Build history of the part. All positions in model axes, mm. Face numbers are marked on the shaded views. Give positions to 0.01 mm unless a question says otherwise; leave off trailing zeros. Order: outer loops, then holes, each group sorted by start corner. A loop starts at its lowest first (then second) coordinate and runs counter-clockwise, first axis right, second up. Notation, with made-up numbers: (65, 12.5) - (111, 12.5) arc R9 ccw to (111, 19.5) - close; hole circle Ø2 at (-23, -24). An arc over 180 degrees is marked (long way). Answer in a Markdown table with one row per item.
```python
from build123d import *

# Parameters (mm, degrees)
F1_DEPTH = 10
F3_DEPTH = 2.5
F4_SIZE  = 1.5
F5_SIZE  = 2.49999
F6_SIZE  = 1
F7_R     = 1.5


# Not quite as in the source:
# - a fillet or chamfer is up to 0.001 mm smaller than in the source, because OpenCascade refuses the exact size


with BuildPart() as f1:
    # F0 (on Top) → F1 (new body, symmetric)
    with BuildSketch(Plane.XY):
        Polygon((63, 0), (-63, 0), (-63, 9), (-66, 9), (-66, -3), (66, -3), (66, 9), (63, 9), align=None)
    extrude(amount=F1_DEPTH, both=True)

    # F2 (on face) → F3 (join)
    with BuildSketch(Plane.XZ.offset(3)):
        with BuildLine():
            ThreePointArc((-18.4661853126, -10), (-21, 0), (-18.4661853126, 10))
            Line((-18.4661853126, 10), (-20.7123151772, 10))
            ThreePointArc((-20.7123151772, 10), (-23, 0), (-20.7123151772, -10))
            Line((-20.7123151772, -10), (-18.4661853126, -10))
        make_face()
        with BuildLine():
            Line((20.7123151772, 10), (18.4661853126, 10))
            ThreePointArc((18.4661853126, 10), (21, 0), (18.4661853126, -10))
            Line((18.4661853126, -10), (20.7123151772, -10))
            ThreePointArc((20.7123151772, -10), (23, 0), (20.7123151772, 10))
        make_face()
    extrude(amount=F3_DEPTH)

    # F4
    f4_edges = [f1.edges().sort_by_distance(p)[0] for p in [
        (-21, -5.5, 0),
        (21, -5.5, 0),
    ]]
    chamfer(f4_edges, length=F4_SIZE)

    # F5 (size 2.5 in the source; OpenCascade refuses exactly that, so slightly less here)
    f5_edges = [f1.edges().sort_by_distance(p)[0] for p in [
        (-23, -3, 0),
        (23, -3, 0),
    ]]
    chamfer(f5_edges, length=F5_SIZE)

    # F6
    f6_edges = [f1.edges().sort_by_distance(p)[0] for p in [
        (-66, -3, 0),
        (66, -3, 0),
    ]]
    chamfer(f6_edges, length=F6_SIZE)

    # F7
    f7_edges = [f1.edges().sort_by_distance(p)[0] for p in [
        (63, 0, 0),
        (-63, 0, 0),
    ]]
    fillet(f7_edges, radius=F7_R)


solid = f1.part
```
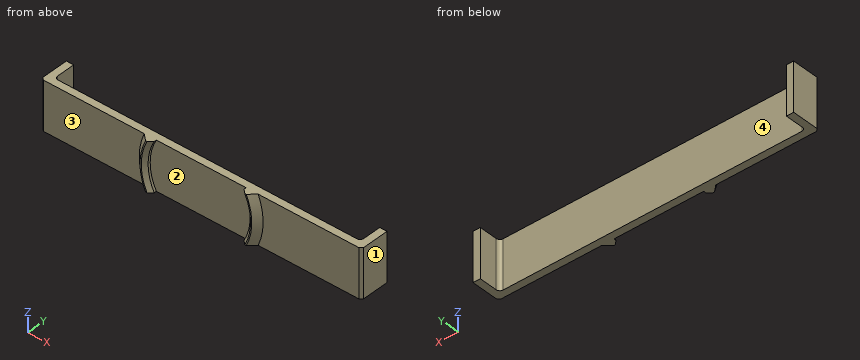
1. Drop flat-ended pins along their axis: P1, Ø1.5, axis at x = 44, z = -8, coming from the -Y side; P2, Ø10, axis at x = -11, z = 4, coming from the +Y side; P3, Ø5, axis at x = 20.5, y = 4.5, coming from the +Z side (1 decimal). Give the stop position or say it passes through.
Check result:
| item | result |
|---|---|
| P1 | stops at y = -3 |
| P2 | stops at y = 0 |
| P3 | passes through |
2. Probe line 1 (X direction, y = 4, z = -1.5); line 2 (Y direction, x = -4, z = -5.75); line 3 (X direction, y = -2.25, z = 3). List the from-to ranges inside material, lowest first.
Check result:
| item | result |
|---|---|
| line 1 | x = -66 to -63, 63 to 66 |
| line 2 | y = -3 to 0 |
| line 3 | x = -65.75 to 65.75 |
3. Cut at B-B on x = -8.5. Write the cut outline in (y, z), and give its area (3 significant figures).
Check result:
| item | result |
|---|---|
| outline | (-3, -10) - (0, -10) - (0, 10) - (-3, 10) - close |
| area | 60.0 mm² |
4. Cut at A-A on y = 6.5. Write the cut outline in (x, z).
Check result:
| item | result |
|---|---|
| outline | (-66, -10) - (-63, -10) - (-63, 10) - (-66, 10) - close; (63, -10) - (66, -10) - (66, 10) - (63, 10) - close |
5. Two-plate mould, pull along X, no slides. Class the marked faces 1, 2, 3 and 4: +X half, -X half, draft (parallel to the pull), parting line (faces both ways), or undercut.
Check result:
| item | result |
|---|---|
| face 1 | +X half |
| face 2 | undercut |
| face 3 | draft |
| face 4 | undercut |
